```python
from build123d import *

# Parameters (mm, degrees)
SKETCH1_R           = 2
BOSS_EXTRUDE1_DEPTH = 11.25
SKETCH3_W           = 0.64
SKETCH3_H           = 0.4


with BuildPart() as part:
    # Sketch1 → Boss-Extrude1 (new, symmetric)
    with BuildSketch(Plane(origin=(0, 0, 0), x_dir=(0, 0, -1), z_dir=(1, 0, 0))):
        with Locations(Location((0, 0, 0), (0, 0, 180))):
            Circle(SKETCH1_R)
    extrude(amount=BOSS_EXTRUDE1_DEPTH, both=True)

    # Sketch3 → Cut-Revolve1 (revolve, cut)
    with BuildSketch(Plane(origin=(0, 0, 0), x_dir=(1, 0, 0), z_dir=(0, 1, 0)), mode=Mode.PRIVATE) as cut_revolve1_sk:
        with Locations((-9.92, 1.8)):
            Rectangle(SKETCH3_W, SKETCH3_H)
    cut_revolve1 = revolve(cut_revolve1_sk.sketch.rotate(Axis((-12.375, 0, 0), (1, 0, 0)), 180), axis=Axis((-12.375, 0, 0), (1, 0, 0)), mode=Mode.SUBTRACT)

    # Mirror1: Cut-Revolve1 across plane
    add(cut_revolve1.mirror(Plane(origin=(0, 0, 0), x_dir=(0, 0, 1), z_dir=(1, 0, 0))), mode=Mode.SUBTRACT)


solid = part.part
```
Verification items for the finished model (mm, model axes). A direction names the side the tool comes from. Coordinates: 2 decimals unless noted, no trailing zeros. Order: outer loops, then holes, each group sorted by start corner. A loop starts at its lowest first (then second) coordinate and runs counter-clockwise, first axis right, second up. Notation, with made-up numbers: (27.5, -8.75) -> (69.5, -8.75) arc R17 ccw to (69.5, 0.25) -> close; hole circle Ø6 at (77.5, 85). An arc over 180 degrees is marked (long way). Put each result on its own line as item: value. Start each with the question number.
1) Cross-section at C-C (z = 0.65). Enter the section's corners in (x, y).
2) Cross-section at A-A (y = -0.6). Enter the section's corners in (x, z), plus the area to 3 significant figures.
3) Cross-section at B-B (x = -7.5). Enter the section's corners in (y, z).
4) Release check for a two-part mould opening along X. For faces 1 (the cylindrical face through (-9.916, -0.481, 1.526)), 2 (the flat face through (11.25, 0, 0)), 3 (the cylindrical face through (-11, 2, 0)) record: pulls with the +X half, pulls with the -X half, needs draft (parallel to the pull), parting line crosses it, or undercut.
5) Material ranges on L1, parallel to X at y = -0.95, z = -1.65; L2, parallel to Y at x = -3.75, z = 0.45; L3, parallel to Y at x = -6.5, z = -0.8, recorded low to high.
6) Tool access check on faces 4 (the cylindrical face through (9.916, -0.481, 1.526)), 5 (the flat face through (-11.25, 0, 0)). Record the directions out of +Z, -Z, +X, -X, +Y, -Y that give a thin tool (end or side, any length) a straight path to the whole face; none if there is none.
Geometry check:
1. outline: (-11.25, -1.89) -> (-10.24, -1.89) -> (-10.24, -1.46) -> (-9.6, -1.46) -> (-9.6, -1.89) -> (9.6, -1.89) -> (9.6, -1.46) -> (10.24, -1.46) -> (10.24, -1.89) -> (11.25, -1.89) -> (11.25, 1.89) -> (10.24, 1.89) -> (10.24, 1.46) -> (9.6, 1.46) -> (9.6, 1.89) -> (-9.6, 1.89) -> (-9.6, 1.46) -> (-10.24, 1.46) -> (-10.24, 1.89) -> (-11.25, 1.89) -> close
2. outline: (-11.25, -1.91) -> (-10.24, -1.91) -> (-10.24, -1.48) -> (-9.6, -1.48) -> (-9.6, -1.91) -> (9.6, -1.91) -> (9.6, -1.48) -> (10.24, -1.48) -> (10.24, -1.91) -> (11.25, -1.91) -> (11.25, 1.91) -> (10.24, 1.91) -> (10.24, 1.48) -> (9.6, 1.48) -> (9.6, 1.91) -> (-9.6, 1.91) -> (-9.6, 1.48) -> (-10.24, 1.48) -> (-10.24, 1.91) -> (-11.25, 1.91) -> close
2. area: 84.8 mm^2
3. outline: circle Ø4 at (0, 0)
4. face 1: undercut
4. face 2: pulls with the +X half
4. face 3: needs draft
5. L1: x = -11.25 to -10.24, -9.6 to 9.6, 10.24 to 11.25
5. L2: y = -1.95 to 1.95
5. L3: y = -1.83 to 1.83
6. face 4: none
6. face 5: +Z, -Z, -X, +Y, -Y
